Geometry check sheet. Reference: the model listing, model coordinates, mm. Face numbers are marked on the shaded views. A direction names the side the tool comes from. Round coordinates to 2 decimals unless told otherwise and drop trailing zeros. Order: outer loops, then holes, each group sorted by start corner. A loop starts at its lowest first (then second) coordinate and runs counter-clockwise, first axis right, second up. Notation, with made-up numbers: (49.5, -34.75) - (69.5, -34.75) arc R9 cw to (69.5, -19.75) - close; hole circle Ø6 at (64, -36). An arc over 180 degrees is marked (long way). Return JSON: item names as keys, results as strings. Group by question number.
Q1. Sectioned sample at A-A, the plane x = -23. Record the cut outline in (y, z).
Q2. Tool access check on the marked faces 1 and 2. Record the directions out of +Z, -Z, +X, -X, +Y, -Y that give a thin tool (end or side, any length) a straight path to the whole face; none if there is none.
Q3. Gauge pin test, flat ends, axial feed: pin 1 Ø2.5 at (x, y) = (0, 0) entering from -Z; pin 2 Ø1 at (y, z) = (10.5, 5) entering from +X; pin 3 Ø3 at (x, z) = (8.5, 4) entering from -Y. Record the tip position at first contact, or that the pin passes through.
Q4. Sectioned sample at B-B, the plane x = -12. Record the cut outline in (y, z), then the cut area to 3 significant figures.
Q5. Material ranges on line 1 along Y through (x, z) = (-22.5, 2.75); line 2 along X through (y, z) = (-12.5, 1.5); line 3 along Y through (x, z) = (-16, 3.75), recorded low to high.
Q6. Sectioned sample at C-C, the plane z = 2. Give the number of separate pieces and of enclosed holes in the cut face, then the cut area to 3 significant figures.
Q7. Sectioned sample at D-D, the plane y = -6. Record the cut outline in (x, z).
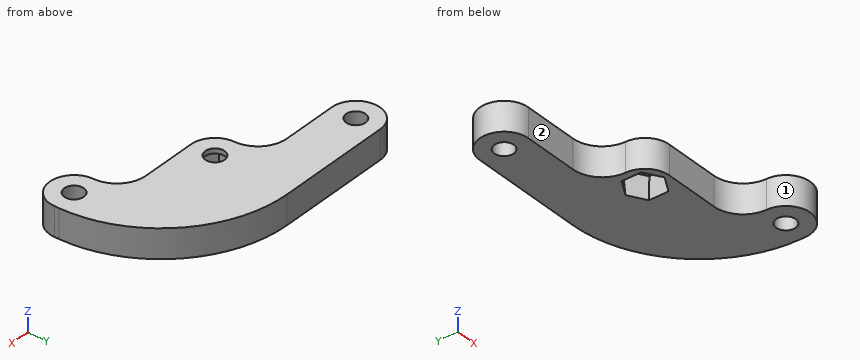
```python
from build123d import *

# Parameters (mm, degrees)
F0_R     = 2
F1_DEPTH = 6
F3_DEPTH = 5
F3_TAPER = -5


with BuildPart() as f1:
    # F0 (on Top) → F1 (new body)
    with BuildSketch(Plane.XY):
        with BuildLine():
            ThreePointArc((-22.4499443206, 16), (-27.4499443206, 11), (-22.4499443206, 6))
            Line((-22.4499443206, 6), (-11, 6))
            ThreePointArc((-11, 6), (-6.7573593129, 4.2426406871), (-5, 0))
            ThreePointArc((-5, 0), (-3.5355339059, -3.5355339059), (0, -5))
            Line((0, -5), (11.4499443206, -5))
            ThreePointArc((11.4499443206, -5), (15.6925850078, -6.7573593129), (17.4499443206, -11))
            ThreePointArc((17.4499443206, -11), (22.4499443206, -16), (27.4499443206, -11))
            Line((27.4499443206, -11), (27.4499443206, -10.047595575))
            ThreePointArc((27.4499443206, -10.047595575), (19.8207802103, 8.3708358897), (1.4023487456, 16))
            Line((1.4023487456, 16), (-22.4499443206, 16))
        make_face()
        with Locations((22.4499443206, -11)):
            Circle(F0_R, mode=Mode.SUBTRACT)
        with Locations((-22.4499443206, 11)):
            Circle(F0_R, mode=Mode.SUBTRACT)
        Circle(F0_R, mode=Mode.SUBTRACT)
    extrude(amount=F1_DEPTH)

    # F2 (on face) → F3 (cut)
    with BuildSketch(Plane(origin=(0, 0, 0), x_dir=(1, 0, 0), z_dir=(0, 0, -1))):
        Polygon((0, -4.0414518843), (3.5, -2.0207259422), (3.5, 2.0207259422), (0, 4.0414518843), (-3.5, 2.0207259422), (-3.5, -2.0207259422), align=None)
    extrude(amount=-F3_DEPTH, taper=F3_TAPER, mode=Mode.SUBTRACT)


solid = f1.part
```
Reply:
{
 "1": {"outline": "(6.03, 0) - (9.08, 0) - (9.08, 6) - (6.03, 6) - close; (12.92, 0) - (15.97, 0) - (15.97, 6) - (12.92, 6) - close"},
 "2": {"face 1": "+Z, -Z, -Y", "face 2": "+Z, -Z, -X, -Y"},
 "3": {"pin 1": "through", "pin 2": "x = 18.03", "pin 3": "y = -5"},
 "4": {"outline": "(6, 0) - (16, 0) - (16, 6) - (6, 6) - close", "area": "60.0 mm^2"},
 "5": {"line 1": "6 to 9, 13 to 16", "line 2": "17.68 to 21.13, 23.77 to 27.22", "line 3": "6 to 16"},
 "6": {"separate pieces": "1", "enclosed holes": "3", "area": "787 mm^2"},
 "7": {"outline": "(14.77, 0) - (27.13, 0) - (27.13, 6) - (14.77, 6) - close"}
}
